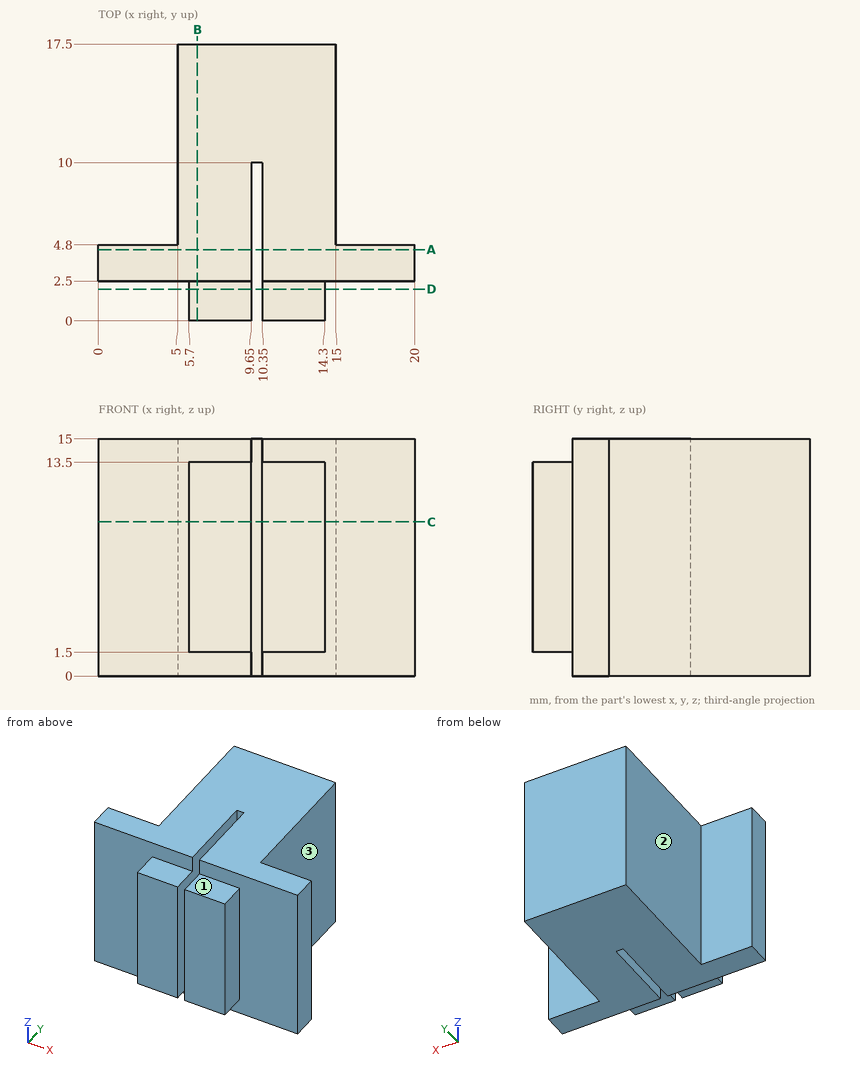
Can you work these out from the drawing? Everything is in mm from the part's minimum corner. A direction names the side the tool comes from. Give positions to 0.01 mm unless a question says otherwise; leave off trailing zeros. Order: outer loops, then holes, each group sorted by start corner. A loop starts at its lowest first (then second) coordinate and runs counter-clockwise, first axis right, second up. Notation, with made-up numbers: M -30,73.5 L 3,73.5 A21 cw 3,107.5 Z; hole C 53.25,62 d6. An arc over 180 degrees is marked long. Use a Markdown table: item, result. Add a question column.
Item 1: Suppose I cut it at D-D (y = 2). List the corners of the cut face in (x, z) for me.
Item 2: Will these pins go through, and if not, where does the flat tip stop? pin 1 (3 mm diameter, centred on y = 13, z = 8, fed in from -X); pin 2 (0.8 mm diameter, centred on x = 12, y = 2, fed in from -Z); pin 3 (1.2 mm diameter, centred on y = 1.5, z = 6.5, fed in from +X).
Item 3: Suppose I cut it at A-A (y = 4.5). List the corners of the cut face in (x, z) for me, then the cut area to 4 significant figures.
Item 4: For the marked faces 1, 2 and 3, which set-ups out of +Z, -Z, +X, -X, +Y, -Y let a thin tool reach every point of the face, with its end or its side?
Item 5: If I drill on L1, parallel to X at y = 9.5, z = 12; L2, parallel to X at y = 1.5, z = 2; L3, parallel to X at y = 13.5, z = 6.5, over which ranges is the centre line in solid material (lowest first)? Write a range as [from, to].
Item 6: Suppose I cut it at B-B (x = 6.25). List the corners of the cut face in (y, z) for me, then the cut area to 3 significant figures.
Item 7: Suppose I cut it at C-C (z = 9.75). List the corners of the cut face in (x, y) for me, then the cut area to 4 significant figures.
Answer sheet:
| question | item | result |
|---|---|---|
| 1 | outline | M 5.7,1.5 L 9.65,1.5 L 9.65,13.5 L 5.7,13.5 Z; M 10.35,1.5 L 14.3,1.5 L 14.3,13.5 L 10.35,13.5 Z |
| 2 | pin 1 | stops at x = 5 |
| 2 | pin 2 | stops at z = 1.5 |
| 2 | pin 3 | stops at x = 14.3 |
| 3 | outline | M 0,0 L 9.65,0 L 9.65,15 L 0,15 Z; M 10.35,0 L 20,0 L 20,15 L 10.35,15 Z |
| 3 | area | 289.5 mm² |
| 4 | face 1 | +Z, +X, -X, -Y |
| 4 | face 2 | +Z, -Z, -X, +Y |
| 4 | face 3 | +Z, -Z, +X, +Y |
| 5 | L1 | x = [5, 9.65], [10.35, 15] |
| 5 | L2 | x = [5.7, 9.65], [10.35, 14.3] |
| 5 | L3 | x = [5, 15] |
| 6 | outline | M 0,1.5 L 2.5,1.5 L 2.5,0 L 17.5,0 L 17.5,15 L 2.5,15 L 2.5,13.5 L 0,13.5 Z |
| 6 | area | 255 mm² |
| 7 | outline | M 0,2.5 L 5.7,2.5 L 5.7,0 L 9.65,0 L 9.65,10 L 10.35,10 L 10.35,0 L 14.3,0 L 14.3,2.5 L 20,2.5 L 20,4.8 L 15,4.8 L 15,17.5 L 5,17.5 L 5,4.8 L 0,4.8 Z |
| 7 | area | 187.5 mm² |
